Source: CAD feature listing. Evaluate the final solid. Frame: model axes, mm. Face numbers are marked on the shaded views. Round coordinates to 2 decimals unless told otherwise and drop trailing zeros. Write each loop counter-clockwise with the first axis right and the second up, starting at its lowest first coordinate (ties: lowest second). Pieces come first, ordered by that corner, then holes. Notation, with made-up numbers: M 30,5.5 L 36,5.5 A14 cw 36,28.5 Z; hole C 50,7 d8. An arc over 180 degrees is marked long. Answer in a Markdown table with one row per item.
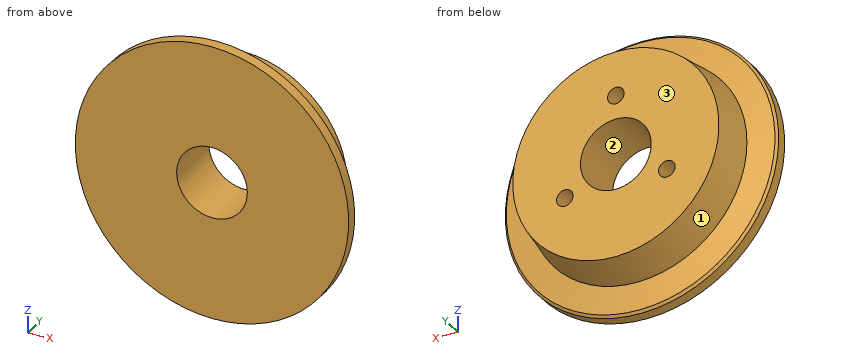
from build123d import *

# Parameters (mm, degrees)
SKETCH_4_R               = 11.6
SKETCH_4_R_2             = 1.1
EXTRUDE_1_DEPTH          = 1.1
EXTRUDE_START            = 1.5
SKETCH_4_3_R             = 9.25
SKETCH_4_3_R_2           = 1.1
EXTRUDE_2_DEPTH          = 3.3
CHAMFER_1_SIZE           = 0.2
SKETCH_6_R               = 3
CUT_EXTRUDE_1_DEPTH      = 18.092688495
SKETCH_7_R               = 0.7
CUT_EXTRUDE_2_DEPTH      = 3
PATTERN_CIRCULAR_1_COUNT = 3
CHAMFER_2_SIZE           = 3.3
CHAMFER_2_SIZE_2         = 0.5


with BuildPart() as part:
    # 草图4 → 凸台-拉伸1 (new body)
    with BuildSketch(Plane(origin=(0, 0, 0), x_dir=(1, 0, 0), z_dir=(0, 1, 0))):
        with Locations(Location((0, 0, 0), (0, 0, 270))):
            Circle(SKETCH_4_R)
        with Locations(Location((0, 0, 0), (0, 0, 270))):
            Circle(SKETCH_4_R_2, mode=Mode.SUBTRACT)
    extrude(amount=EXTRUDE_1_DEPTH)

    # 倒角1
    chamfer_1_edges = [part.edges().sort_by_distance(p)[0] for p in [
        (0, 1.1, -11.6),
    ]]
    chamfer(chamfer_1_edges, length=CHAMFER_1_SIZE)


with BuildPart() as body_2:
    # 草图4<3> → 凸台-拉伸2 (new body)
    with BuildSketch(Plane(origin=(0, 0, 0), x_dir=(1, 0, 0), z_dir=(0, 1, 0)).offset(EXTRUDE_START)):
        with Locations(Location((0, 0, 0), (0, 0, 270))):
            Circle(SKETCH_4_3_R)
        with Locations(Location((0, 0, 0), (0, 0, 270))):
            Circle(SKETCH_4_3_R_2, mode=Mode.SUBTRACT)
    extrude(amount=EXTRUDE_2_DEPTH)


    add(part.part)  # loft_1 joins it to this body
    # loft up to a face of the part (loft_1)
    loft([Face(Wire([body_2.edges().sort_by_distance((-6.742959804, 1.5, -6.33206073))[0]])), Face(Wire([body_2.edges().sort_by_distance((8.310242353, 1.1, -7.803837008))[0]]))])

    # 草图6 → 切除-拉伸1 (cut, through all)
    with BuildSketch(Plane(origin=(0, 4.8, 0), x_dir=(1, 0, 0), z_dir=(0, 1, 0))):
        with Locations(Location((0, 0, 0), (0, 0, 270))):
            Circle(SKETCH_6_R)
    extrude(amount=-CUT_EXTRUDE_1_DEPTH, mode=Mode.SUBTRACT)

    # 草图7 → 切除-拉伸2 (cut)
    with BuildSketch(Plane(origin=(0, 4.8, 0), x_dir=(1, 0, 0), z_dir=(0, 1, 0))):
        with Locations(Location((0, -5, 0), (0, 0, 270))):
            Circle(SKETCH_7_R)
    cut_extrude_2 = extrude(amount=-CUT_EXTRUDE_2_DEPTH, mode=Mode.SUBTRACT)

    # 阵列(圆周)1: 切除-拉伸2 ×3 about axis
    pattern_circular_1_axis = Axis((0, 0, 0), (0, 1, 0))
    for i in range(1, PATTERN_CIRCULAR_1_COUNT):
        add(cut_extrude_2.rotate(pattern_circular_1_axis, i * 360 / PATTERN_CIRCULAR_1_COUNT), mode=Mode.SUBTRACT)

    # 倒角2
    # the kernel refuses this chamfer: 3.3, 0.5 mm, written as the material it takes off along each edge
    with BuildSketch(Plane(origin=(0, 4.8, 0), x_dir=(0, 0, 1), z_dir=(-1, 0, 0))) as chamfer_2_piece_1:
        Polygon((9.25, -CHAMFER_2_SIZE), (9.25 - CHAMFER_2_SIZE_2, 0), (9.25, 0), align=None)
    revolve(axis=Axis((0, 4.8, 0), (0, 1, 0)), mode=Mode.SUBTRACT)


solid = body_2.part
Q1. Contact query for a flat-ended pin moving along its axis: pin 1 Ø1.6 at (x, z) = (-4.33, -2.5) entering from -Y. Output: stop coordinate, or through.
Solutions:
| item | result |
|---|---|
| pin 1 | stops at y = 0 |
Q2. Pull-direction query (X, two-part tool) for the marked faces 1, 2 and 3; classes: pulls with the +X half, pulls with the -X half, needs draft (parallel to the pull), parting line crosses it, or undercut.
Solutions:
| item | result |
|---|---|
| face 1 | parting line crosses it |
| face 2 | undercut |
| face 3 | needs draft |
Q3. Material intervals for probe 1 along X at (y, z) = (3.65, -2.5); probe 2 along Z at (x, y) = (-0.5, 3.2); probe 3 along X at (y, z) = (4.1, -2.5), sorted ascending.
Solutions:
| item | result |
|---|---|
| probe 1 | x = -8.57 to -5.03, -3.63 to -1.66, 1.66 to 3.63, 5.03 to 8.57 |
| probe 2 | z = -8.98 to -2.96, 2.96 to 4.51, 5.49 to 8.98 |
| probe 3 | x = -8.5 to -5.03, -3.63 to -1.66, 1.66 to 3.63, 5.03 to 8.5 |
Q4. Section A-A (y = 2.1). Return loops of the section in (x, z).
Solutions:
| item | result |
|---|---|
| outline | C 0,0 d18.32; hole C -4.33,-2.5 d1.4; hole C 0,0 d6; hole C 0,5 d1.4; hole C 4.33,-2.5 d1.4 |
Q5. Section B-B (y = 3.3). Return loops of the section in (x, z), and give its area (3 significant figures).
Solutions:
| item | result |
|---|---|
| outline | C 0,0 d17.95; hole C -4.33,-2.5 d1.4; hole C 0,0 d6; hole C 0,5 d1.4; hole C 4.33,-2.5 d1.4 |
| area | 220 mm2 |
